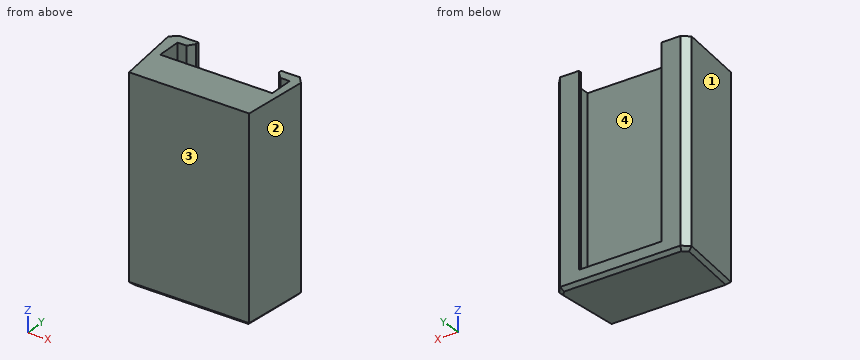
```python
from build123d import *

# Parameters (mm, degrees)
BOSS_EXTRUDE1_DEPTH = 30
BOSS_EXTRUDE2_DEPTH = 2
CHAMFER8_SIZE       = 0.5


with BuildPart() as part:
    # Sketch1 → Boss-Extrude1 (new body)
    with BuildSketch(Plane.XY):
        Polygon((-17.075998832, -1.699461634), (0.924001168, -1.699461634), (1.706939946, 8.236405705), (0.797202797, 9.300538366), (-2.002797203, 9.300538366), (-2.002797203, 8.800538366), (-1.025998832, 7.800538366), (0.324001168, 7.800538366), (0.324001168, 4.100538366), (-16.475998832, 4.100538366), (-16.475998832, 7.800538366), (-15.125998832, 7.800538366), (-14.402797203, 8.800538366), (-14.402797203, 9.300538366), (-17.202797203, 9.300538366), (-18.292206063, 8.421227081), align=None)
    extrude(amount=-BOSS_EXTRUDE1_DEPTH)

    # Sketch2 → Boss-Extrude2 (add)
    with BuildSketch(Plane(origin=(0, 0, -30), x_dir=(-1, 0, 0), z_dir=(0, 0, -1))):
        Polygon((2.002797203, 9.300538366), (14.402797203, 9.300538366), (16.475998832, 9.300538366), (16.475998832, 4.100538366), (-0.324001168, 4.100538366), (-0.324001168, 9.300538366), align=None)
    extrude(amount=-BOSS_EXTRUDE2_DEPTH)

    # Chamfer8
    chamfer8_edges = [part.edges().sort_by_distance(p)[0] for p in [
        (1.315470557, 3.268472036, -30),
        (1.252071371, 8.768472036, -30),
        (-8.202797203, 9.300538366, -30),
        (-17.684102447, 3.360882724, -30),
        (-17.747501633, 8.860882724, -30),
        (-8.075998832, -1.699461634, -30),
    ]]
    chamfer(chamfer8_edges, length=CHAMFER8_SIZE)


solid = part.part
```
Read the model definition and answer for the solid it produces. Units are mm, in the model's axes. Face numbers are marked on the shaded views. Give positions to 0.01 mm unless a question says otherwise; leave off trailing zeros. Write each loop counter-clockwise with the first axis right and the second up, starting at its lowest first coordinate (ties: lowest second). Pieces come first, ordered by that corner, then holes. Notation, with made-up numbers: (9.5, -3) - (14.5, -3) arc R24 ccw to (14.5, 18) - close; hole circle Ø9 at (44, 47.25). An arc over 180 degrees is marked (long way). Write item = value, one per line. Start each with the question number.
Item 1: Find section A-A (x = -13.5). Give the vertices of the cut face in (y, z).
Item 2: The mould has two halves that part along X. Classify the marked faces 1, 2, 3 and 4: +X half, -X half, draft (parallel to the pull), parting line (faces both ways), or undercut.
Item 3: Find the intervals of material crossed by probe 1 along Y at (x, z) = (-0.25, -10); probe 2 along Y at (x, z) = (-8.5, -12.5); probe 3 along Z at (x, y) = (-9.75, 5.5), in increasing order. Write a range as [from, to].
Item 4: Each of these flat-tipped pins is pushed along its axis until it touches: P1, Ø5, axis at x = -7.5, z = -19, coming from the +Y side; P2, Ø3, axis at y = 0.5, z = -22, coming from the +X side; P3, Ø4, axis at y = 6, z = -19, coming from the +X side; P4, Ø6, axis at x = -14, z = -10.5, coming from the +Y side. Where does it stop, or does it pass through?
Item 5: Find section D-D (x = -16). Give the vertices of the cut face in (y, z), then the cut area to 3 significant figures.
Item 6: Find section B-B (z = -22). Give the vertices of the cut face in (x, y), then the cut area to 3 significant figures.
Item 7: Find section C-C (y = 0.25). Give the vertices of the cut face in (x, z).
Response:
q1.outline = (-1.7, -29.5) - (-1.2, -30) - (8.8, -30) - (9.3, -29.5) - (9.3, -28) - (4.1, -28) - (4.1, 0) - (-1.7, 0) - close
q2.face_1 = -X half
q2.face_2 = +X half
q2.face_3 = draft
q2.face_4 = undercut
q3.probe_1 = [-1.7, 4.1], [7.8, 9.3]
q3.probe_2 = [-1.7, 4.1]
q3.probe_3 = [-30, -28]
q4.P1 = 4.1
q4.P2 = 1.22
q4.P3 = 1.69
q4.P4 = 9.3
q5.outline = (-1.7, -29.5) - (-1.2, -30) - (8.8, -30) - (9.3, -29.5) - (9.3, 0) - (7.8, 0) - (7.8, -28) - (4.1, -28) - (4.1, 0) - (-1.7, 0) - close
q5.area = 226 mm²
q6.outline = (-18.29, 8.42) - (-17.08, -1.7) - (0.92, -1.7) - (1.71, 8.24) - (0.8, 9.3) - (-2, 9.3) - (-2, 8.8) - (-1.03, 7.8) - (0.32, 7.8) - (0.32, 4.1) - (-16.48, 4.1) - (-16.48, 7.8) - (-15.13, 7.8) - (-14.4, 8.8) - (-14.4, 9.3) - (-17.2, 9.3) - close
q6.area = 127 mm²
q7.outline = (-17.31, -29.5) - (-16.81, -30) - (0.58, -30) - (1.08, -29.5) - (1.08, 0) - (-17.31, 0) - close
